Source: CAD feature listing. Evaluate the final solid. Frame: model axes, mm. A direction names the side the tool comes from. Give positions to 0.01 mm unless a question says otherwise; leave off trailing zeros. Loops run counter-clockwise (first coordinate to the right, second up) from the corner with the lowest first, then second, coordinate; pieces in that order, holes last. Notation, with made-up numbers: (47, 81.5) -> (59, 81.5) arc R20 ccw to (59, 107.5) -> close; hole circle Ø11 at (69, 74). An arc over 180 degrees is marked (long way). Return JSON: item names as keys, results as strings. Group by question number.
(1) Access query for faces 1 (the face through (52, 10, -25)), 2 (the face through (53, 20, -3)), 3 (the face through (5, 17, -47)). Directions: +Z, -Z, +X, -X, +Y, -Y. A direction counts if a zero-diameter tool reaches every point of the face in a straight line with its end or side. Return the directions, or none.
(2) Ray query, line 1 (X direction, y = 4.3, z = -25); line 2 (Y direction, x = 5, z = -2.5); line 3 (Z direction, x = -12.5, y = 4). Return the intervals inside material, ascending. Write a range as from..to.
(3) Cut plane C-C on x = 61. Return loops of the section in (y, z).
(4) Cut plane D-D on x = -12.5. Return loops of the section in (y, z).
(5) Cut plane B-B on z = -25. Return loops of the section in (x, y), then the cut area to 3 significant figures.
(6) Cut plane A-A on x = 5. Return loops of the section in (y, z).
(7) Draft query along Z for faces 4 (the face through (-12.728, 5.028, -26.735)), 5 (the face through (-12, 7, -25)), 6 (the face through (5, 22.2, -5)), 7 (the face through (2, 16, -25)). Return one class per face: released by +Z, released by -Z, zero draft, split by the parting line, or undercut.
(8) Pin query (flat end, axial travel): pin 1 (10 mm diameter, centred on x = 28, y = 14, fed in from +Z); pin 2 (1.5 mm diameter, centred on x = 34, z = -46.5, fed in from +Y); pin 3 (1.5 mm diameter, centred on y = 17, z = -13.5, fed in from -X); pin 4 (1 mm diameter, centred on x = -12.5, z = -24.5, fed in from +Y). Return the tip coordinate at first contact, or that it passes through.
```python
from build123d import *

# Parameters (mm, degrees)
SKETCH1_W           = 100
SKETCH1_H           = 50
BOSS_EXTRUDE1_DEPTH = 20
SKETCH4_W           = 25
SKETCH4_H           = 7
CUT_EXTRUDE1_DEPTH  = 100
SKETCH5_R           = 4.5
SKETCH5_R_2         = 1.75
CUT_EXTRUDE2_DEPTH  = 4
FILLET2_R           = 1.5
SKETCH6_R           = 3
SKETCH6_R_2         = 2
BOSS_EXTRUDE3_DEPTH = 5
CUT_EXTRUDE3_DEPTH  = 10
SKETCH10_R          = 3
CUT_EXTRUDE4_DEPTH  = 10
CUT_EXTRUDE5_DEPTH  = 54
BOSS_EXTRUDE4_DEPTH = 50


with BuildPart() as part:
    # Sketch1 → Boss-Extrude1 (new body)
    with BuildSketch(Plane(origin=(0, 0, 0), x_dir=(1, 0, 0), z_dir=(0, 1, 0))):
        with Locations((50, 25)):
            Rectangle(SKETCH1_W, SKETCH1_H)
    extrude(amount=BOSS_EXTRUDE1_DEPTH)

    # Sketch4 → Revolve1 (revolve)
    with BuildSketch(Plane.ZY):
        with Locations((-12.5, 3.5)):
            Rectangle(SKETCH4_W, SKETCH4_H)
    revolve(axis=Axis((0, 0, -25), (0, 1, 0)))

    # Sketch2 → Cut-Extrude1 (cut)
    with BuildSketch(Plane(origin=(100, 0, 0), x_dir=(0, 0, -1), z_dir=(1, 0, 0))):
        with BuildLine():
            Line((45, 20), (5, 20))
            ThreePointArc((5, 20), (25, 10), (45, 20))
        make_face()
    extrude(amount=-CUT_EXTRUDE1_DEPTH, mode=Mode.SUBTRACT)

    # Sketch5 → Cut-Extrude2 (cut)
    with BuildSketch(Plane(origin=(0, 7, 0), x_dir=(1, 0, 0), z_dir=(0, 1, 0))):
        with Locations((-12.5, 25)):
            Circle(SKETCH5_R)
        with Locations((-12.5, 25)):
            Circle(SKETCH5_R_2, mode=Mode.SUBTRACT)
    extrude(amount=-CUT_EXTRUDE2_DEPTH, mode=Mode.SUBTRACT)

    # Fillet2
    fillet2_edges = [part.edges().sort_by_distance(p)[0] for p in [
        (-17, 7, -25),
    ]]
    fillet(fillet2_edges, radius=FILLET2_R)

    # Sketch6 → Boss-Extrude3 (add)
    with BuildSketch(Plane.XY):
        with Locations((5, 20)):
            Circle(SKETCH6_R)
        with Locations((5, 20)):
            Circle(SKETCH6_R_2, mode=Mode.SUBTRACT)
    extrude(amount=-BOSS_EXTRUDE3_DEPTH)

    # Sketch8 → Cut-Extrude3 (cut)
    with BuildSketch(Plane.XY):
        with BuildLine():
            Line((3, 20), (7, 20))
            ThreePointArc((7, 20), (5, 18), (3, 20))
        make_face()
    extrude(amount=-CUT_EXTRUDE3_DEPTH, mode=Mode.SUBTRACT)

    # Sketch10 → Cut-Extrude4 (cut)
    with BuildSketch(Plane(origin=(0, 0, -50), x_dir=(-1, 0, 0), z_dir=(0, 0, -1))):
        with Locations((-5, 20)):
            Circle(SKETCH10_R)
    extrude(amount=-CUT_EXTRUDE4_DEPTH, mode=Mode.SUBTRACT)

    # Sketch11 → Cut-Extrude5 (cut)
    with BuildSketch(Plane(origin=(0, 0, -50), x_dir=(-1, 0, 0), z_dir=(0, 0, -1))):
        Polygon((-2, 20), (0, 18.845299462), (0, 20), align=None)
    extrude(amount=-CUT_EXTRUDE5_DEPTH, mode=Mode.SUBTRACT)

    # Sketch12 → Boss-Extrude4 (add)
    with BuildSketch(Plane(origin=(0, 0, -50), x_dir=(-1, 0, 0), z_dir=(0, 0, -1))):
        Polygon((-2, 20), (-2, 0), (0, 0), (0, 18.845299462), align=None)
    extrude(amount=-BOSS_EXTRUDE4_DEPTH)


solid = part.part
```
Answers:
{
 "1": {"face 1": "+X, +Y", "face 2": "+Z, -Z, +X, +Y", "face 3": "-Z, +Y"},
 "2": {"line 1": "-25..-17, -14.25..-10.75, -8..100", "line 2": "0..18, 22..23", "line 3": "-46.65..-29.5, -26.75..-23.25, -20.5..-3.35"},
 "3": {"outline": "(0, -50) -> (20, -50) -> (20, -45) arc R25 cw to (20, -5) -> (20, 0) -> (0, 0) -> close"},
 "4": {"outline": "(0, -46.65) -> (7, -46.65) -> (7, -31) arc R1.5 ccw to (5.5, -29.5) -> (3, -29.5) -> (3, -26.75) -> (7, -26.75) -> (7, -23.25) -> (3, -23.25) -> (3, -20.5) -> (5.5, -20.5) arc R1.5 ccw to (7, -19) -> (7, -3.35) -> (0, -3.35) -> close"},
 "5": {"outline": "(-25, 0) -> (100, 0) -> (100, 10) -> (2, 10) -> (2, 20) -> (0, 18.85) -> (0, 7) -> (-6.5, 7) arc R1.5 ccw to (-8, 5.5) -> (-8, 3) -> (-10.75, 3) -> (-10.75, 7) -> (-14.25, 7) -> (-14.25, 3) -> (-17, 3) -> (-17, 5.5) arc R1.5 ccw to (-18.5, 7) -> (-25, 7) -> close", "area": "1,170 mm²"},
 "6": {"outline": "(0, -50) -> (17, -50) -> (17, -42.35) arc R25 cw to (18, -6.67) -> (18, 0) -> (0, 0) -> close; (22, -5) -> (23, -5) -> (23, 0) -> (22, 0) -> close"},
 "7": {"face 4": "undercut", "face 5": "zero draft", "face 6": "released by -Z", "face 7": "undercut"},
 "8": {"pin 1": "z = 0", "pin 2": "y = 20", "pin 3": "x = 0", "pin 4": "y = 7"}
}
